Here's the drawing with two shaded views (mm, measured from the low corner). I have some questions. A direction names the side the tool comes from. Give positions to 0.01 mm unless a question says otherwise; leave off trailing zeros. Loops run counter-clockwise (first coordinate to the right, second up) from the corner with the lowest first, then second, coordinate; pieces in that order, holes last. Notation, with made-up numbers: M 58,27 L 117,27 A30 cw 117,54 Z; hole C 38.5,41.25 d2. An arc over 180 degrees is marked long. Write item = value, one per line. Start each with the question number.
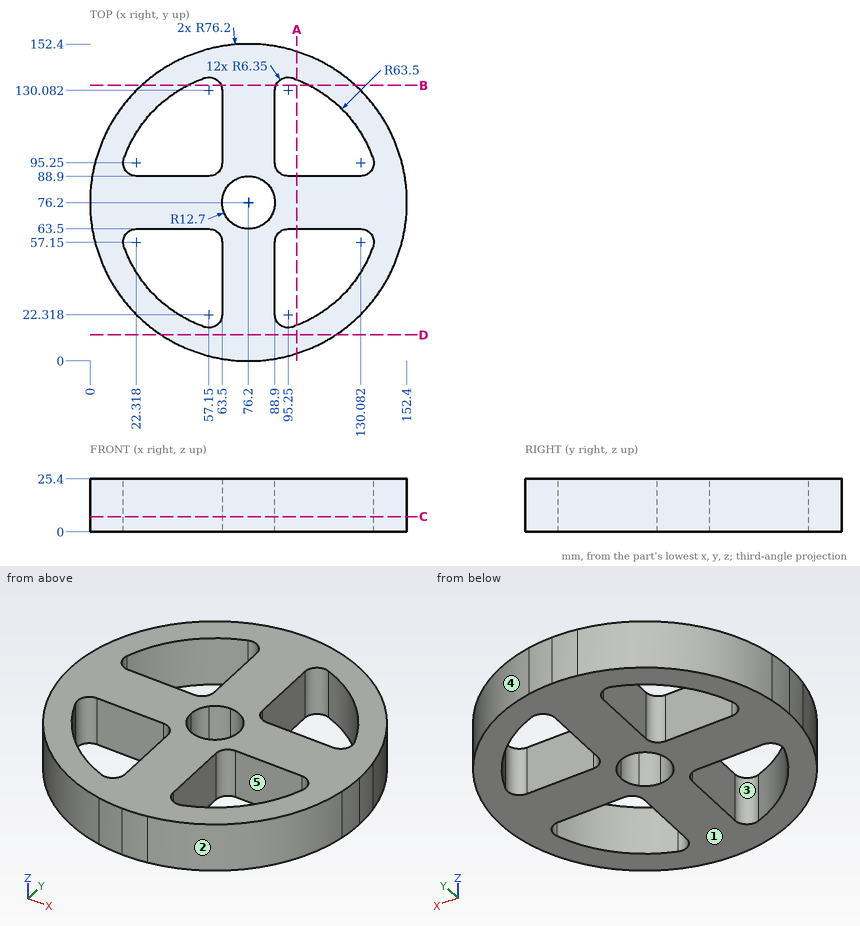
Q1. If we section it at C-C, the plane z = 7.25: State how many separate pieces and enclosed holes the cut face has, then the cut area to 3 significant figures.
Q2. Will these pins go through, and if not, where does the flat tip stop? pin 1 (3 mm diameter, centred on y = 110.5, z = 8.5, fed in from +X); pin 2 (1 mm diameter, centred on y = 28, z = 8, fed in from +X) (1 decimal); pin 3 (7.5 mm diameter, centred on x = 45.5, z = 11, fed in from +Y) (1 decimal); pin 4 (6 mm diameter, centred on x = 90.5, y = 40.5, fed in from -Z).
Q3. If we section it at B-B, the plane y = 132.5: List the corners of the cut face in (x, z) for me, then the cut area to 3 significant figures.
Q4. If we section it at A-A, the plane x = 99.5: List the corners of the cut face in (y, z) for me, then the cut area to 3 significant figures.
Q5. On a 3-axis mill with a long thin cutter (end or side, diameter ignored), from which of +Z, -Z, +X, -X, +Y, -Y can I reach the whole of each face in a straight line? I mean the marked faces 4 and 5. Say none if no direction works.
Q6. If I drill on line 1 along X through (y, z) = (110, 18) (1 decimal); line 2 along X through (y, z) = (126, 2.75) (1 decimal); line 3 along Y through (x, z) = (36, 21.5) (1 decimal), over which ranges is the centre line in solid material (lowest first)?
Q7. We'd pull the mould along Y, two halves only. Please class the marked faces 1, 2 and 3: pulls with the +Y half, pulls with the -Y half, needs draft (parallel to the pull), parting line crosses it, or undercut.
Q8. If we section it at D-D, the plane y = 12.5: List the corners of the cut face in (x, z) for me, then the cut area to 3 significant figures.
Resolved:
q1.separate_pieces = 1
q1.enclosed_holes = 5
q1.area = 11,000 mm²
q2.pin_1 = 144.98
q2.pin_2 = 135.6
q2.pin_3 = 147.5
q2.pin_4 = 0
q3.outline = M 24.85,0 L 46.83,0 L 46.83,25.4 L 24.85,25.4 Z; M 63.02,0 L 89.38,0 L 89.38,25.4 L 63.02,25.4 Z; M 105.57,0 L 127.55,0 L 127.55,25.4 L 105.57,25.4 Z
q3.area = 1,790 mm²
q4.outline = M 3.65,0 L 17.13,0 L 17.13,25.4 L 3.65,25.4 Z; M 63.5,0 L 88.9,0 L 88.9,25.4 L 63.5,25.4 Z; M 135.27,0 L 148.75,0 L 148.75,25.4 L 135.27,25.4 Z
q4.area = 1,330 mm²
q5.face_4 = +Z, -Z, +X, +Y
q5.face_5 = +Z, -Z
q6.line_1 = 7.9 to 22.4, 63.5 to 88.9, 130 to 144.5
q6.line_2 = 18.5 to 36.8, 63.5 to 88.9, 115.6 to 133.9
q6.line_3 = 11.5 to 27, 63.5 to 88.9, 125.4 to 140.9
q7.face_1 = needs draft
q7.face_2 = pulls with the -Y half
q7.face_3 = undercut
q8.outline = M 34.38,0 L 118.02,0 L 118.02,25.4 L 34.38,25.4 Z
q8.area = 2,120 mm²
